Read the model definition and answer for the solid it produces. Units are mm, in the model's axes. A direction names the side the tool comes from. Coordinates: 2 decimals unless noted, no trailing zeros. Write each loop counter-clockwise with the first axis right and the second up, starting at its lowest first coordinate (ties: lowest second). Pieces come first, ordered by that corner, then holes.
1) Each of these flat-tipped pins is pushed along its axis until it touches: pin 1 Ø5 at (y, z) = (157, -0.5) entering from +X; pin 2 Ø8 at (x, z) = (0, 0) entering from +Y; pin 3 Ø6 at (x, z) = (19.05, 0) entering from -Y (3 decimals). Where does it stop, or does it pass through?
2) Which of the six approach directions +Z, -Z, +X, -X, +Y, -Y give full straight-line access (tool end or side, diameter ignored) to faces 4 (the face through (-23.29, 63.39, 2.55)), 5 (the face through (0, 3.175, 0)), 6 (the face through (-17.169, 181.099, -1.725)), 7 (the face through (-2.48, 107.788, 0.111)), 8 (the face through (41.1, 12.7, 5.4))?
3) The part is cut by section B-B (y = 92.5). Determine the outline of the cut face in (x, z), then the cut area to 3 significant figures.
4) Determine the mould class of faces 1 (the face through (-50.8, 6, 0)), 2 (the face through (-13.39, 146.76, -0.11)), 3 (the face through (35, 0, 0)) for opening direction X: +X half, -X half, draft (parallel to the pull), parting line (faces both ways), or undercut.
5) The part is cut by section A-A (y = 149.86). Give the number of separate pieces and of enclosed holes in the cut face, then the cut area to 3 significant figures.
6) Find the intervals of material crossed by line 1 (X direction, y = 149.86, z = -4.5) (3 decimals); line 2 (Y direction, x = 22, z = 0) (3 decimals); line 3 (X direction, y = 177.5, z = 1.75), in increasing order.
from build123d import *

# Parameters (mm, degrees)
SKETCH1_W                        = 101.6
SKETCH1_H                        = 15.875
BOSS_EXTRUDE1_DEPTH              = 190.5
CUT_EXTRUDE1_REACH               = 199.795
SKETCH2_W                        = 19.05
SKETCH2_H                        = 177.8
CUT_EXTRUDE2_REACH               = 199.795
SKETCH4_W                        = 50.8
SKETCH4_H                        = 3.175
F_3_8_CLEARANCE_HOLE1_D          = 10.0838
F_3_8_CLEARANCE_HOLE1_DEPTH      = 38.608
F_3_8_CLEARANCE_HOLE1_TIP        = 3.029479155
F_1_4_0_25_DIAMETER_HOLE2_D      = 6.35
CUT_EXTRUDE3_REACH               = 199.795
SKETCH11_R                       = 19.05
F_1_4_20_TAPPED_HOLE2_D          = 5.1054
F_1_4_20_TAPPED_HOLE2_DEPTH      = 18.542
F_1_4_20_TAPPED_HOLE2_TIP        = 1.533816902
LPATTERN1_COUNT                  = 2
LPATTERN1_PITCH                  = 12.7
F_1_4_0_25_DIAMETER_HOLE1_D      = 6.35
F_1_4_0_25_DIAMETER_HOLE1_DEPTH  = 38.608
F_1_4_0_25_DIAMETER_HOLE1_TIP    = 1.907732465
F_1_4_20_TAPPED_HOLE3_AT_2_COUNT = 2
F_1_4_20_TAPPED_HOLE3_AT_2_PITCH = 50.8
CUT_EXTRUDE4_REACH               = 199.795
SKETCH19_R                       = 6.35
MIRROR3_COPY_1_D                 = 6.35


with BuildPart() as part:
    # Sketch1 → Boss-Extrude1 (new body)
    with BuildSketch(Plane(origin=(0, 0, 0), x_dir=(1, 0, 0), z_dir=(0, 1, 0))):
        Rectangle(SKETCH1_W, SKETCH1_H)
    extrude(amount=BOSS_EXTRUDE1_DEPTH)

    # Sketch2 → Cut-Extrude1 (cut, up to next)
    with BuildSketch(Plane.XY.offset(7.9375), mode=Mode.PRIVATE) as cut_extrude1_sk1:
        with Locations((-41.275, 101.6)):
            Rectangle(SKETCH2_W, SKETCH2_H)
    cut_extrude1_tool1 = extrude(cut_extrude1_sk1.sketch, amount=-CUT_EXTRUDE1_REACH, mode=Mode.PRIVATE) & part.part
    # Sketch2 → Cut-Extrude1 (cut, up to next)
    with BuildSketch(Plane.XY.offset(7.9375), mode=Mode.PRIVATE) as cut_extrude1_sk2:
        with Locations((41.275, 101.6)):
            Rectangle(SKETCH2_W, SKETCH2_H)
    cut_extrude1_tool2 = extrude(cut_extrude1_sk2.sketch, amount=-CUT_EXTRUDE1_REACH, mode=Mode.PRIVATE) & part.part
    add(cut_extrude1_tool1.solids().sort_by_distance((-41.275, 101.6, 7.9375))[0], mode=Mode.SUBTRACT)
    add(cut_extrude1_tool2.solids().sort_by_distance((41.275, 101.6, 7.9375))[0], mode=Mode.SUBTRACT)

    # Sketch4 → Cut-Extrude2 (cut, up to next)
    with BuildSketch(Plane.XY.offset(7.9375), mode=Mode.PRIVATE) as cut_extrude2_sk1:
        with Locations((0, 1.5875)):
            Rectangle(SKETCH4_W, SKETCH4_H)
    cut_extrude2_tool1 = extrude(cut_extrude2_sk1.sketch, amount=-CUT_EXTRUDE2_REACH, mode=Mode.PRIVATE) & part.part
    add(cut_extrude2_tool1.solids().sort_by_distance((0, 1.5875, 7.9375))[0], mode=Mode.SUBTRACT)

    # 3/8 Clearance Hole1
    with Locations(Plane(origin=(0, 12.7, 0), x_dir=(-1, 0, 0), z_dir=(0, 1, 0))):
        with Locations((41.275, 0), (-41.275, 0)):
            Hole(F_3_8_CLEARANCE_HOLE1_D / 2, depth=F_3_8_CLEARANCE_HOLE1_DEPTH)
            with Locations((0, 0, -(F_3_8_CLEARANCE_HOLE1_DEPTH + F_3_8_CLEARANCE_HOLE1_TIP / 2))):  # 118° drill point
                Cone(0, F_3_8_CLEARANCE_HOLE1_D / 2, F_3_8_CLEARANCE_HOLE1_TIP, mode=Mode.SUBTRACT)

    # 1/4 (0.25) Diameter Hole2 (through all)
    with Locations(Plane.XY.offset(7.9375)):
        with Locations((12.7, 149.86), (25.4, 149.86)):
            f_1_4_0_25_diameter_hole2 = Hole(F_1_4_0_25_DIAMETER_HOLE2_D / 2)

    # Sketch11 → Cut-Extrude3 (cut, up to next)
    with BuildSketch(Plane.XY.offset(7.9375), mode=Mode.PRIVATE) as cut_extrude3_sk1:
        with Locations((0, 88.9)):
            Circle(SKETCH11_R)
    cut_extrude3_tool1 = extrude(cut_extrude3_sk1.sketch, amount=-CUT_EXTRUDE3_REACH, mode=Mode.PRIVATE) & part.part
    add(cut_extrude3_tool1.solids().sort_by_distance((0, 88.9, 7.9375))[0], mode=Mode.SUBTRACT)

    # 1/4-20 Tapped Hole2
    with Locations(Plane(origin=(0, 190.5, 0), x_dir=(1, 0, 0), z_dir=(0, 1, 0))):
        with Locations((-19.05, 0), (19.05, 0), (0, 0)):
            Hole(F_1_4_20_TAPPED_HOLE2_D / 2, depth=F_1_4_20_TAPPED_HOLE2_DEPTH)
            with Locations((0, 0, -(F_1_4_20_TAPPED_HOLE2_DEPTH + F_1_4_20_TAPPED_HOLE2_TIP / 2))):  # 118° drill point
                Cone(0, F_1_4_20_TAPPED_HOLE2_D / 2, F_1_4_20_TAPPED_HOLE2_TIP, mode=Mode.SUBTRACT)

    # LPattern1: 1/4 (0.25) Diameter Hole2 ×2
    with Locations(*[(0, i * LPATTERN1_PITCH, 0) for i in range(1, LPATTERN1_COUNT)]):
        add(f_1_4_0_25_diameter_hole2, mode=Mode.SUBTRACT)

    # 1/4 (0.25) Diameter Hole1
    with Locations(Plane.XY.offset(7.9375)):
        with Locations((-12.7, 63.5), (12.7, 63.5)):
            Hole(F_1_4_0_25_DIAMETER_HOLE1_D / 2, depth=F_1_4_0_25_DIAMETER_HOLE1_DEPTH)
            with Locations((0, 0, -(F_1_4_0_25_DIAMETER_HOLE1_DEPTH + F_1_4_0_25_DIAMETER_HOLE1_TIP / 2))):  # 118° drill point
                Cone(0, F_1_4_0_25_DIAMETER_HOLE1_D / 2, F_1_4_0_25_DIAMETER_HOLE1_TIP, mode=Mode.SUBTRACT)

    # Sketch17 → 1/4-20 Tapped Hole3 (revolve, cut)
    with BuildSketch(Plane(origin=(31.75, 114.3, 0), x_dir=(0, 0, -1), z_dir=(0, 1, 0))):
        Polygon((0, 0), (0, 20.075816902), (2.5527, 18.542), (2.5527, 0), align=None)
    f_1_4_20_tapped_hole3 = revolve(axis=Axis((38.1, 114.3, 0), (-1, 0, 0)), mode=Mode.SUBTRACT)

    # 1/4-20 Tapped Hole3 at 2: 1/4-20 Tapped Hole3 ×2
    with Locations(*[(0, -i * F_1_4_20_TAPPED_HOLE3_AT_2_PITCH, 0) for i in range(1, F_1_4_20_TAPPED_HOLE3_AT_2_COUNT)]):
        add(f_1_4_20_tapped_hole3, mode=Mode.SUBTRACT)

    # Mirror2: 1/4-20 Tapped Hole3 across plane
    add(f_1_4_20_tapped_hole3.mirror(Plane(origin=(0, 0, 0), x_dir=(0, 0, 1), z_dir=(1, 0, 0))), mode=Mode.SUBTRACT)

    # Mirror2 copy 1 sketch → Mirror2 copy 1 (revolve, cut)
    with BuildSketch(Plane(origin=(-31.75, 63.5, 0), x_dir=(0, 0, -1), z_dir=(0, 1, 0))):
        Polygon((0, 0), (0, -20.075816902), (2.5527, -18.542), (2.5527, 0), align=None)
    revolve(axis=Axis((-38.1, 63.5, 0), (-1, 0, 0)), mode=Mode.SUBTRACT)

    # Sketch19 → Cut-Extrude4 (cut, up to next)
    with BuildSketch(Plane.XY.offset(7.9375), mode=Mode.PRIVATE) as cut_extrude4_sk1:
        with Locations((0, 139.7)):
            Circle(SKETCH19_R)
    cut_extrude4_tool1 = extrude(cut_extrude4_sk1.sketch, amount=-CUT_EXTRUDE4_REACH, mode=Mode.PRIVATE) & part.part
    add(cut_extrude4_tool1.solids().sort_by_distance((0, 139.7, 7.9375))[0], mode=Mode.SUBTRACT)

    # Mirror3: 1/4 (0.25) Diameter Hole2 across plane
    add(f_1_4_0_25_diameter_hole2.mirror(Plane(origin=(0, 0, 0), x_dir=(0, 0, 1), z_dir=(1, 0, 0))), mode=Mode.SUBTRACT)

    # Mirror3 copy 1 (through all)
    with Locations(Plane(origin=(0, 12.7, 7.9375), x_dir=(-1, 0, 0), z_dir=(0, 0, 1))):
        with Locations((12.7, -149.86), (25.4, -149.86)):
            Hole(MIRROR3_COPY_1_D / 2)


solid = part.part
Reported:
1. pin 1: stops at x = 31.75
1. pin 2: stops at y = 190.5
1. pin 3: stops at y = 3.175
2. face 4: -X
2. face 5: +Z, -Z, -Y
2. face 6: +Y
2. face 7: +Z, -Z
2. face 8: +Z, -Z, +X, +Y
3. outline: (-31.75, -7.94) - (-18.71, -7.94) - (-18.71, 7.94) - (-31.75, 7.94) - close; (18.71, -7.94) - (31.75, -7.94) - (31.75, 7.94) - (18.71, 7.94) - close
3. area: 414 mm2
4. face 1: -X half
4. face 2: undercut
4. face 3: draft
5. separate pieces: 5
5. enclosed holes: 0
5. area: 605 mm2
6. line 1: x = -31.75 to -28.575, -22.225 to -15.875, -9.525 to 9.525, 15.875 to 22.225, 28.575 to 31.75
6. line 2: y = 3.175 to 60.947, 66.053 to 111.747, 116.853 to 190.5
6. line 3: x = -31.75 to -20.91, -17.19 to -1.86, 1.86 to 17.19, 20.91 to 31.75
